Geometry check sheet. Reference: the model listing, model coordinates, mm. A direction names the side the tool comes from. Round coordinates to 2 decimals unless told otherwise and drop trailing zeros. Order: outer loops, then holes, each group sorted by start corner. A loop starts at its lowest first (then second) coordinate and runs counter-clockwise, first axis right, second up. Notation, with made-up numbers: M -18.75,-30.75 L 25.25,-30.75 A21 cw 25.25,8.25 Z; hole C 19,38 d8. An arc over 180 degrees is marked long. Return JSON: item names as keys, results as strings. Group by question number.
```python
from build123d import *

# Parameters (mm, degrees)
SKETCH1_R           = 6.375
BOSS_EXTRUDE1_DEPTH = 15
SKETCH9_R           = 7.75
BOSS_EXTRUDE5_DEPTH = 15
SKETCH10_R          = 5.25
CUT_EXTRUDE4_DEPTH  = 5
SKETCH11_R          = 5.25
CUT_EXTRUDE5_DEPTH  = 10
CUT_EXTRUDE5_DRAFT  = -20
SKETCH12_R          = 3.875
CUT_EXTRUDE6_DEPTH  = 30


with BuildPart() as part:
    # Sketch1 → Boss-Extrude1 (new body)
    with BuildSketch(Plane(origin=(0, 0, 0), x_dir=(1, 0, 0), z_dir=(0, 1, 0))):
        with Locations(Location((0, 0, 0), (0, 0, 270))):
            Circle(SKETCH1_R)
    extrude(amount=BOSS_EXTRUDE1_DEPTH)

    # Sketch9 → Boss-Extrude5 (add)
    with BuildSketch(Plane(origin=(0, 15, 0), x_dir=(1, 0, 0), z_dir=(0, 1, 0))):
        with Locations(Location((0, 0, 0), (0, 0, 270))):
            Circle(SKETCH9_R)
    extrude(amount=BOSS_EXTRUDE5_DEPTH)

    # Sketch10 → Cut-Extrude4 (cut)
    with BuildSketch(Plane(origin=(0, 30, 0), x_dir=(1, 0, 0), z_dir=(0, 1, 0))):
        with Locations(Location((0, 0, 0), (0, 0, 270))):
            Circle(SKETCH10_R)
    extrude(amount=-CUT_EXTRUDE4_DEPTH, mode=Mode.SUBTRACT)


with BuildPart() as cut_extrude5_tool:
    # Sketch11 → Cut-Extrude5 (with draft: the straight prism first)
    with BuildSketch(Plane(origin=(0, 25, 0), x_dir=(1, 0, 0), z_dir=(0, 1, 0))):
        with Locations(Location((0, 0, 0), (0, 0, 270))):
            Circle(SKETCH11_R)
    extrude(amount=-CUT_EXTRUDE5_DEPTH)
    # Cut-Extrude5: the draft: its side faces are tilted about the plane it starts from
    cut_extrude5_sides = [cut_extrude5_tool.faces().sort_by_distance(p)[0] for p in [
        (0, 20, -5.25),
    ]]
    draft(cut_extrude5_sides, Plane(origin=(0, 25, 0), x_dir=(1, 0, 0), z_dir=(0, 1, 0)), CUT_EXTRUDE5_DRAFT)


with BuildPart() as part_1:
    add(part.part)

    # Cut-Extrude5: cut by cut_extrude5_tool
    add(cut_extrude5_tool.part, mode=Mode.SUBTRACT)

    # Sketch12 → Cut-Extrude6 (cut)
    with BuildSketch(Plane.XZ):
        with Locations(Location((0, 0, 0), (0, 0, 270))):
            Circle(SKETCH12_R)
    extrude(amount=-CUT_EXTRUDE6_DEPTH, mode=Mode.SUBTRACT)


solid = part_1.part
```
Q1. Section check A-A on x = 0. Record the cut outline in (y, z) (3 decimals).
Q2. Material ranges on line 1 along X through (y, z) = (26.5, 0); line 2 along Y through (x, z) = (6.75, -3.25); line 3 along Z through (x, y) = (3.25, 19.75), recorded low to high.
Q3. Section check B-B on z = 0. Record the cut outline in (x, y) (3 decimals), plus the area to 3 significant figures.
Q4. Section check C-C on y = 19.5. Record the cut outline in (x, z) (3 decimals).
Q5. Release check for a two-part mould opening along X. For faces 3 (the face through (-6, 15, -3)), 4 (the face through (3.842, 10.463, 0.504)), 5 (the face through (-6.223, 7.395, -1.382)) record: +X half, -X half, draft (parallel to the pull), parting line (faces both ways), or undercut.
Q6. Set-up check for faces 1 (the face through (1.6, 27.5, 5)), 2 (the face through (-3, 0, 3)): record each of +Z, -Z, +X, -X, +Y, -Y from which the full face is reachable in a straight line by a thin tool's end or side.
Q7. Section check D-D on y = 27.75. Record the cut outline in (x, z).
Q8. Depth check by flat-ended pin: pin 1 Ø6 at (y, z) = (23, 2.5) entering from +X; pin 2 Ø1 at (x, y) = (-5.5, 19.5) entering from +Z; pin 3 Ø6 at (x, z) = (0, 0) entering from -Y; pin 4 Ø8 at (x, y) = (-5.5, 22) entering from -Z. Enter the tip coordinate at first touch or a pass-through.
Geometry check:
{
 "1": {"outline": "M 0,-6.375 L 15,-6.375 L 15,-7.75 L 30,-7.75 L 30,-5.25 L 25,-5.25 L 21.222,-3.875 L 0,-3.875 Z; M 0,3.875 L 21.222,3.875 L 25,5.25 L 30,5.25 L 30,7.75 L 15,7.75 L 15,6.375 L 0,6.375 Z"},
 "2": {"line 1": "x = -7.75 to -5.25, 5.25 to 7.75", "line 2": "y = 15 to 30", "line 3": "z = -7.04 to -2.11, 2.11 to 7.04"},
 "3": {"outline": "M -7.75,15 L -6.375,15 L -6.375,0 L -3.875,0 L -3.875,21.222 L -5.25,25 L -5.25,30 L -7.75,30 Z; M 3.875,0 L 6.375,0 L 6.375,15 L 7.75,15 L 7.75,30 L 5.25,30 L 5.25,25 L 3.875,21.222 Z", "area": "172 mm^2"},
 "4": {"outline": "C 0,0 d15.5; hole C 0,0 d7.75"},
 "5": {"face 3": "draft", "face 4": "undercut", "face 5": "parting line"},
 "6": {"face 1": "+Y", "face 2": "+Z, -Z, +X, -X, -Y"},
 "7": {"outline": "C 0,0 d15.5; hole C 0,0 d10.5"},
 "8": {"pin 1": "stops at x = 7.75", "pin 2": "stops at z = 5.92", "pin 3": "passes through", "pin 4": "stops at z = -7.6"}
}
